from build123d import *

# Parameters (mm, degrees)
BOX002_W      = 156
BOX002_H      = 72
BOX002_DEPTH  = 8
BOX001_W      = 10
BOX001_H      = 52
BOX001_DEPTH  = 10
BOX_W         = 160
BOX_H         = 72
BOX_DEPTH     = 10
SKETCH_R      = 1.65
HOLE_DEPTH    = 160.001
SKETCH001_R   = 1.65
HOLE001_DEPTH = 10.001


with BuildPart() as obj1:
    # Box002 → Box002 (new body)
    with BuildSketch(Plane(origin=(2, 0, 0), x_dir=(1, 0, 0), z_dir=(0, 0, 1))):
        with Locations((78, 36)):
            Rectangle(BOX002_W, BOX002_H)
    extrude(amount=BOX002_DEPTH)


with BuildPart() as obj2:
    # Box001 → Box001 (new body)
    with BuildSketch(Plane(origin=(0, 10, 0), x_dir=(1, 0, 0), z_dir=(0, 0, 1))):
        with Locations((5, 26)):
            Rectangle(BOX001_W, BOX001_H)
    extrude(amount=BOX001_DEPTH)


with BuildPart() as part_mirroring:
    # Part__Mirroring: instance of obj2
    add(obj2.part.mirror(Plane(origin=(80, 0, 0), x_dir=(0, -1, 0), z_dir=(1, 0, 0))))


with BuildPart() as body:
    # Box → Box (new body)
    with BuildSketch(Plane.XY):
        with Locations((80, 36)):
            Rectangle(BOX_W, BOX_H)
    extrude(amount=BOX_DEPTH)

    # Cut: cut obj2
    add(obj2.part, mode=Mode.SUBTRACT)

    # Cut001: cut Part__Mirroring
    add(part_mirroring.part, mode=Mode.SUBTRACT)

    # Cut002: cut obj1
    add(obj1.part, mode=Mode.SUBTRACT)

    # Sketch (on Face1 of BaseFeature) → Hole (cut, through all)
    with BuildSketch(Plane(origin=(0, 0, 0), x_dir=(0, -1, 0), z_dir=(-1, 0, 0))):
        with Locations((-5, 4)):
            Circle(SKETCH_R)
        with Locations((-67, 4)):
            Circle(SKETCH_R)
    extrude(amount=-HOLE_DEPTH, mode=Mode.SUBTRACT)

    # Sketch001 (on Face2 of Hole) → Hole001 (cut, through all)
    with BuildSketch(Plane.XY.offset(10)):
        with Locations((37, 20)):
            Circle(SKETCH001_R)
        with Locations((37, 52)):
            Circle(SKETCH001_R)
        with Locations((64, 52)):
            Circle(SKETCH001_R)
        with Locations((64, 20)):
            Circle(SKETCH001_R)
        with Locations((117, 47)):
            Circle(SKETCH001_R)
        with Locations((117, 7)):
            Circle(SKETCH001_R)
    extrude(amount=-HOLE001_DEPTH, mode=Mode.SUBTRACT)


solid = body.part
The model under review builds one solid part; all positions refer to its coordinate system, in mm. A direction names the side the tool comes from. Give positions to 0.01 mm unless a question says otherwise; leave off trailing zeros. Write each loop counter-clockwise with the first axis right and the second up, starting at its lowest first coordinate (ties: lowest second). Pieces come first, ordered by that corner, then holes.
1. For P1, Ø2, axis at y = 25, z = 9, coming from the -X side; P2, Ø4.5, axis at x = 37, y = 20, coming from the -Z side; P3, Ø1.6, axis at y = 47.5, z = 9.5, coming from the +X side; P4, Ø1.5, axis at x = 45.5, z = 5.5, coming from the -Y side, all flat-tipped, find the tip position at first contact; note any pin that passes through.
2. Add section A-A, the plane y = 52. Write out the cut boundary in (x, z).
3. Add section D-D, the plane x = 81. Write out the cut boundary in (y, z), plus the area to 3 significant figures.
4. Draft analysis for pull direction X (two halves, no side actions). For faces 1 (the flat face through (2, 5, 6)), 2 (the flat face through (158.4, 62, 7.2)), 3 (the flat face through (0, 67, 6)), 4 (the cylindrical face through (62.35, 52.07, 9.01)), state which applies: +X half, -X half, draft (parallel to the pull), parting line (faces both ways), or undercut.
5. Add section C-C, the plane y = 67. Write out the cut boundary in (x, z).
6. Add section B-B, the plane x = 117. Write out the cut boundary in (y, z), plus the area to 3 significant figures.
7. Wall thickness on L1, parallel to X at y = 67.5, z = 1; L2, parallel to Y at x = 37, z = 8.6; L3, parallel to Z at x = 1.1, y = 5: over which ranges is each line inside the solid? List them lowest first.
8. Tool access review of faces 5 (the flat face through (158, 5, 6)), 6 (the cylindrical face through (62.35, 20.07, 9.01)), 7 (the flat face through (158.4, 10, 7.2)), 8 (the flat face through (0, 5, 6)), 9 (the flat face through (1.6, 62, 7.2)): name each direction out of +Z, -Z, +X, -X, +Y, -Y from which nothing blocks a thin tool from reaching the whole face with its end or side.
Worked answers:
1. P1: stops at x = 10
1. P2: stops at z = 8
1. P3: stops at x = 150
1. P4: passes through
2. outline: (10, 8) - (35.35, 8) - (35.35, 10) - (10, 10) - close; (38.65, 8) - (62.35, 8) - (62.35, 10) - (38.65, 10) - close; (65.65, 8) - (150, 8) - (150, 10) - (65.65, 10) - close
3. outline: (0, 8) - (72, 8) - (72, 10) - (0, 10) - close
3. area: 144 mm2
4. face 1: undercut
4. face 2: draft
4. face 3: -X half
4. face 4: undercut
5. outline: (0, 0) - (2, 0) - (2, 2.35) - (0, 2.35) - close; (0, 5.65) - (2, 5.65) - (2, 8) - (158, 8) - (158, 5.65) - (160, 5.65) - (160, 10) - (0, 10) - close; (158, 0) - (160, 0) - (160, 2.35) - (158, 2.35) - close
6. outline: (0, 8) - (5.35, 8) - (5.35, 10) - (0, 10) - close; (8.65, 8) - (45.35, 8) - (45.35, 10) - (8.65, 10) - close; (48.65, 8) - (72, 8) - (72, 10) - (48.65, 10) - close
6. area: 131 mm2
7. L1: x = 0 to 2, 158 to 160
7. L2: y = 0 to 18.35, 21.65 to 50.35, 53.65 to 72
7. L3: z = 0 to 2.35, 5.65 to 10
8. face 5: -Z, +Y, -Y
8. face 6: +Z, -Z
8. face 7: +Z, -Z, +X
8. face 8: +Z, -Z, -X, +Y, -Y
8. face 9: +Z, -Z, -X
